Work out the finished part from the listing and answer in its coordinate system (mm). Face numbers are marked on the shaded views. A direction names the side the tool comes from. Give positions to 0.01 mm unless a question says otherwise; leave off trailing zeros. Loops run counter-clockwise (first coordinate to the right, second up) from the corner with the lowest first, then second, coordinate; pieces in that order, holes last. Notation, with made-up numbers: (-24, -35.5) - (35, -35.5) arc R16 cw to (35, -27.5) - close; hole circle Ø4 at (67, 46.5). An arc over 180 degrees is marked (long way). One line per question, with ' | ' between items. Start each with the question number.
1. Which of the six approach directions +Z, -Z, +X, -X, +Y, -Y give full straight-line access (tool end or side, diameter ignored) to the marked faces 1 and 2?
2. Find the intervals of material crossed by line 1 (Z direction, x = 4, y = -12.5); line 2 (X direction, y = 0, z = -6), in increasing order.
3. Each of these flat-tipped pins is pushed along its axis until it touches: pin 1 (10 mm diameter, centred on x = 5.5, z = -5.5, fed in from +Y); pin 2 (8.5 mm diameter, centred on x = 0, y = 0, fed in from +Z); pin 3 (5 mm diameter, centred on y = -11, z = -6.5, fed in from -X); pin 4 (1 mm diameter, centred on x = -2.5, z = 8.5, fed in from -Y). Where does it stop, or does it pass through?
4. For a pull along Z with two mould halves and no side action, classify the marked faces 3, 4, 5 and 6 as released by +Z, released by -Z, zero draft, split by the parting line, or undercut.
5. Section D-D (y = -8.5) is taken. Determine the outline of the cut face in (x, z), plus the area to 3 significant figures.
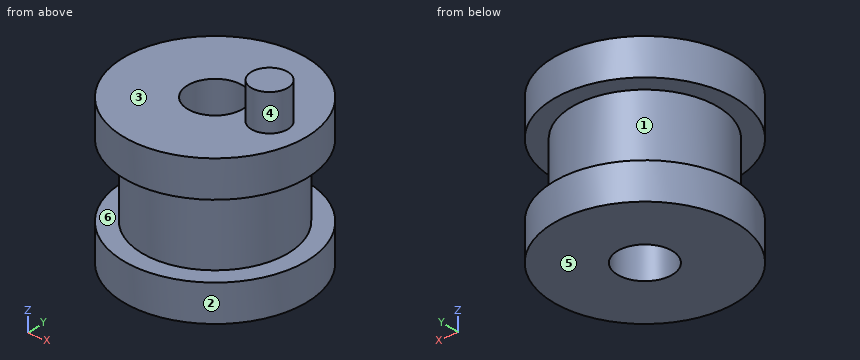
from build123d import *

# Parameters (mm, degrees)
F0_W     = 7.9375
F0_H     = 12.7
F2_R     = 3.175
F3_DEPTH = 6.35


with BuildPart() as f1:
    # F0 (on Front) → F1 (revolve)
    with BuildSketch(Plane.XZ):
        Polygon((4.7625, 12.7), (4.7625, 6.35), (12.7, 6.35), (15.875, 6.35), (15.875, 12.7), align=None)
        with Locations((8.73125, 0)):
            Rectangle(F0_W, F0_H)
        Polygon((12.7, -6.35), (4.7625, -6.35), (4.7625, -12.7), (15.875, -12.7), (15.875, -6.35), align=None)
    revolve(axis=Axis((0, 0, 0), (0, 0, -1)))

    # F2 (on face) → F3 (join)
    with BuildSketch(Plane.XY.offset(12.7)):
        with Locations((9.525, 0)):
            Circle(F2_R)
    extrude(amount=F3_DEPTH)


solid = f1.part
Conclusion:
1) face 1: none | face 2: +Z, -Z
2) line 1: -12.7 to -6.35, 6.35 to 12.7 | line 2: -12.7 to -4.76, 4.76 to 12.7
3) pin 1: y = 15.86 | pin 2: through | pin 3: x = -13.41 | pin 4: y = -15.75
4) face 3: released by +Z | face 4: zero draft | face 5: released by -Z | face 6: undercut
5) outline: (-13.41, -12.7) - (13.41, -12.7) - (13.41, -6.35) - (9.44, -6.35) - (9.44, 6.35) - (13.41, 6.35) - (13.41, 12.7) - (-13.41, 12.7) - (-13.41, 6.35) - (-9.44, 6.35) - (-9.44, -6.35) - (-13.41, -6.35) - close | area: 580 mm²
